The listing builds one solid part. Answer for the finished solid, in the listing's coordinates (mm). A direction names the side the tool comes from. Coordinates: 2 decimals unless noted, no trailing zeros. Order: outer loops, then holes, each group sorted by start corner. A loop starts at its lowest first (then second) coordinate and runs counter-clockwise, first axis right, second up.
from build123d import *

# Parameters (mm, degrees)
SKETCH1_R               = 5
BOSS_EXTRUDE1_DEPTH     = 6
FILLET1_R               = 3
SKETCH2_R               = 1.6
CUT_EXTRUDE1_DEPTH      = 36.846896658
CUT_EXTRUDE2_DEPTH      = 29.930952283
CUT_EXTRUDE2_DEPTH_BACK = 29.930952283
CUT_EXTRUDE3_DEPTH      = 29.460498942
FILLET3_R               = 1
SKETCH5_R               = 1.6
CUT_EXTRUDE4_DEPTH      = 29.460498942
SKETCH6_R               = 3
CUT_EXTRUDE5_DEPTH      = 2
BOSS_EXTRUDE2_START     = -0.5
SKETCH7_R               = 1.6
BOSS_EXTRUDE2_DEPTH     = 0.5


with BuildPart() as part:
    # Sketch1 → Boss-Extrude1 (new body)
    with BuildSketch(Plane(origin=(0, 0, 0), x_dir=(1, 0, 0), z_dir=(0, 1, 0))):
        with BuildLine():
            Line((0, 8), (-17, 8))
            Line((-17, 8), (-17, 15))
            Line((-17, 15), (-24, 15))
            Line((-24, 15), (-24, -15))
            Line((-24, -15), (-17, -15))
            Line((-17, -15), (-17, -8))
            Line((-17, -8), (0, -8))
            ThreePointArc((0, -8), (8, 0), (0, 8))
        make_face()
        with Locations(Location((0, 0, 0), (0, 0, 270))):
            Circle(SKETCH1_R, mode=Mode.SUBTRACT)
    extrude(amount=BOSS_EXTRUDE1_DEPTH)

    # Fillet1
    fillet1_edges = [part.edges().sort_by_distance(p)[0] for p in [
        (-20.5, 0, -15),
        (-20.5, 6, -15),
        (-20.5, 0, 15),
        (-20.5, 6, 15),
    ]]
    fillet(fillet1_edges, radius=FILLET1_R - 0.0001)  # a hair under: the kernel refuses the full size

    # Sketch2 → Cut-Extrude1 (cut, through all)
    with BuildSketch(Plane.ZY.offset(24)):
        with Locations((-12, 3)):
            Circle(SKETCH2_R)
        with Locations((12, 3)):
            Circle(SKETCH2_R)
    extrude(amount=-CUT_EXTRUDE1_DEPTH, mode=Mode.SUBTRACT)

    # Sketch3 → Cut-Extrude2 (cut, two sides: drawn at the far end of the back side and taken through both)
    with BuildSketch(Plane.XY.offset(-CUT_EXTRUDE2_DEPTH_BACK)):
        Polygon((-17, 6), (8, 6), (8, 3), (0, 3), align=None)
    extrude(amount=CUT_EXTRUDE2_DEPTH + CUT_EXTRUDE2_DEPTH_BACK, mode=Mode.SUBTRACT)

    # Sketch4 → Cut-Extrude3 (cut, through all)
    with BuildSketch(Plane(origin=(0, 3, 0), x_dir=(1, 0, 0), z_dir=(0, 1, 0))):
        with BuildLine():
            Line((0, -6), (-16.5, -6))
            ThreePointArc((-16.5, -6), (-22.5, 0), (-16.5, 6))
            Line((-16.5, 6), (0, 6))
            ThreePointArc((0, 6), (6, 0), (0, -6))
        make_face()
    extrude(amount=CUT_EXTRUDE3_DEPTH, mode=Mode.SUBTRACT)

    # Fillet3
    fillet3_edges = [part.edges().sort_by_distance(p)[0] for p in [
        (-17, 3, -8),
        (-17, 3, 8),
    ]]
    fillet(fillet3_edges, radius=FILLET3_R)

    # Sketch5 → Cut-Extrude4 (cut, through all)
    with BuildSketch(Plane(origin=(0, 3, 0), x_dir=(1, 0, 0), z_dir=(0, 1, 0))):
        with Locations(Location((-9, 0, 0), (0, 0, 180))):
            Circle(SKETCH5_R)
        with Locations(Location((-17, 0, 0), (0, 0, 180))):
            Circle(SKETCH5_R)
    extrude(amount=-CUT_EXTRUDE4_DEPTH, mode=Mode.SUBTRACT)

    # Sketch6 → Cut-Extrude5 (cut)
    with BuildSketch(Plane.XZ):
        with Locations(Location((-17, 0, 0), (0, 0, 270))):
            Circle(SKETCH6_R)
        with Locations(Location((-9, 0, 0), (0, 0, 270))):
            Circle(SKETCH6_R)
    extrude(amount=-CUT_EXTRUDE5_DEPTH, mode=Mode.SUBTRACT)

    # Sketch7 → Boss-Extrude2 (add)
    with BuildSketch(Plane.XZ.offset(-2).offset(BOSS_EXTRUDE2_START)):
        with Locations(Location((-17, 0, 0), (0, 0, 180))):
            Circle(SKETCH7_R)
        with Locations(Location((-9, 0, 0), (0, 0, 180))):
            Circle(SKETCH7_R)
    extrude(amount=BOSS_EXTRUDE2_DEPTH)


solid = part.part
(1) Given pin 1 Ø0.9 at (x, y) = (-4.5, 4) entering from +Z; pin 2 Ø1.8 at (y, z) = (2.5, -10.5) entering from +X; pin 3 Ø1.8 at (x, z) = (-18.5, 1) entering from -Y; pin 4 Ø11.5 at (x, z) = (0, 0) entering from -Y, each flat-ended and moving along its own axis, determine where each tip first touches the part or whether it passes through.
(2) A tool of negligible diameter and unlimited length cuts with its end or side. For faces 4 (the flat face through (-17, 4.3, 10.7)), 5 (the cylindrical face through (-22.5, 4.5, 0.1)), 6 (the cylindrical face through (-19.93, 0.99, 0.65)), 7 (the flat face through (-17, 4.3, -10.6)), from which of +Z, -Z, +X, -X, +Y, -Y can it reach the whole face along a straight path? Write none if from no direction.
(3) Find section D-D on y = 0.75. Determine the outline of the cut face in (x, z), then the cut area to 3 significant figures.
(4) Find section A-A on z = -12.5. Determine the outline of the cut face in (x, y).
(5) Find the intervals of material crossed by probe 1 along X at (y, z) = (2.7, 0); probe 2 along X at (y, z) = (0.55, 0); probe 3 along Z at (x, y) = (-14, 5), in increasing order.
(6) Find section C-C on x = -9. Determine the outline of the cut face in (y, z).
(7) The mould has two halves that part along Z. Classify faces 1 (the cylindrical face through (-20.55, 3.07, -13.6)), 2 (the cylindrical face through (8, 1, 0)), 3 (the flat face through (-8.38, 4.48, -7.18)): pulls with the +Z half, pulls with the -Z half, needs draft (parallel to the pull), parting line crosses it, or undercut.
(8) Find section B-B on y = 3.5. Determine the outline of the cut face in (x, z).
Resolved:
1. pin 1: stops at z = 8
1. pin 2: stops at x = -17
1. pin 3: stops at y = 2
1. pin 4: stops at y = 0
2. face 4: +Z, +X, +Y, -Y
2. face 5: +X, +Y
2. face 6: -Y
2. face 7: -Z, +X, +Y, -Y
3. outline: (-24, -13.98) - (-17, -13.98) - (-17, -9) arc R1 cw to (-16, -8) - (0, -8) arc R8 ccw to (0, 8) - (-16, 8) arc R1 cw to (-17, 9) - (-17, 13.98) - (-24, 13.98) - close; hole circle Ø6 at (-17, 0); hole circle Ø6 at (-9, 0); hole circle Ø10 at (0, 0)
3. area: 434 mm2
4. outline: (-24, 0.04) - (-17, 0.04) - (-17, 1.48) - (-24, 1.48) - close; (-24, 4.52) - (-17, 4.52) - (-17, 5.96) - (-24, 5.96) - close
5. probe 1: x = -24 to -18.6, -15.4 to -10.6, -7.4 to -5, 5 to 8
5. probe 2: x = -24 to -20, -14 to -12, -6 to -5, 5 to 8
5. probe 3: z = -8 to -6, 6 to 8
6. outline: (0, -8) - (4.59, -8) - (4.59, -6) - (3, -6) - (3, -1.6) - (2.5, -1.6) - (2.5, 1.6) - (3, 1.6) - (3, 6) - (4.59, 6) - (4.59, 8) - (0, 8) - (0, 3) - (2, 3) - (2, -3) - (0, -3) - close
7. face 1: undercut
7. face 2: parting line crosses it
7. face 3: needs draft
8. outline: (-24, -14.96) - (-17, -14.96) - (-17, -13.52) - (-24, -13.52) - close; (-24, -10.48) - (-17, -10.48) - (-17, -9) arc R1 cw to (-16, -8) - (-2.83, -8) - (-2.83, -6) - (-16.5, -6) arc R6 cw to (-16.5, 6) - (-2.83, 6) - (-2.83, 8) - (-16, 8) arc R1 cw to (-17, 9) - (-17, 10.48) - (-24, 10.48) - close; (-24, 13.52) - (-17, 13.52) - (-17, 14.96) - (-24, 14.96) - close
